Source: CAD feature listing. Evaluate the final solid. Frame: model axes, mm. Round coordinates to 2 decimals unless told otherwise and drop trailing zeros. Order: outer loops, then holes, each group sorted by start corner. A loop starts at its lowest first (then second) coordinate and runs counter-clockwise, first axis right, second up. Notation, with made-up numbers: (78.5, 47) -> (87.5, 47) arc R14 ccw to (87.5, 74) -> close; hole circle Ø11 at (86.5, -7). An arc over 180 degrees is marked (long way). Use a Markdown table: item, result. Add a question column.
```python
from build123d import *

# Parameters (mm, degrees)
SKETCH2_R           = 2.5
SKETCH2_R_2         = 2
BOSS_EXTRUDE1_DEPTH = 10
SKETCH4_R           = 1.5
CUT_EXTRUDE3_DEPTH  = 16


with BuildPart() as part:
    # Sketch2 → Boss-Extrude1 (new body)
    with BuildSketch(Plane(origin=(0, 0, 0), x_dir=(1, 0, 0), z_dir=(0, 1, 0))):
        with BuildLine():
            Line((0, 7.5), (100, 7.5))
            ThreePointArc((100, 7.5), (107.5, 0), (100, -7.5))
            Line((100, -7.5), (0, -7.5))
            ThreePointArc((0, -7.5), (-7.5, 0), (0, 7.5))
        make_face()
        Circle(SKETCH2_R, mode=Mode.SUBTRACT)
        with Locations((100, 0)):
            Circle(SKETCH2_R_2, mode=Mode.SUBTRACT)
    extrude(amount=BOSS_EXTRUDE1_DEPTH)

    # Sketch4 → Cut-Extrude3 (cut, through all)
    with BuildSketch(Plane(origin=(0, 0, -7.5), x_dir=(-1, 0, 0), z_dir=(0, 0, -1))):
        with Locations((0, 5)):
            Circle(SKETCH4_R)
    extrude(amount=-CUT_EXTRUDE3_DEPTH, mode=Mode.SUBTRACT)


solid = part.part
```
1) Section D-D on z = 5. Output: boundary loops of the cut face in (x, y), then the cut area to 3 significant figures.
2) Section C-C on z = -4.5. Output: boundary loops of the cut face in (x, y).
3) Draft query along Z for faces 1 (the cylindrical face through (1.5, 5.07, -4.79)), 2 (the cylindrical face through (-7.5, 4.93, 0.16)), 3 (the cylindrical face through (2.31, 4.93, 0.96)). Return one class per face: pulls with the +Z half, pulls with the -Z half, needs draft (parallel to the pull), parting line crosses it, or undercut.
4) Section B-B on y = 5. Output: boundary loops of the cut face in (x, z), then the cut area to 3 significant figures.
5) Section A-A on z = 0. Output: boundary loops of the cut face in (x, y).
6) Line query: probe 1 along X at (y, z) = (5, 0); probe 2 along Z at (x, y) = (100, 7.75); probe 3 along Y at (x, z) = (0, 5.3). Output: solid intervals per line, ascending. Write a range as from..to.
7) First-contact query: pin 1 Ø1 at (y, z) = (2, -2) entering from +X; pin 2 Ø4 at (y, z) = (4, -5.5) entering from +X; pin 3 Ø1 at (y, z) = (5, 3) entering from +X. Flat tips, straight axial feed; report the tip coordinate or a pass-through.
Conclusion:
| question | item | result |
|---|---|---|
| 1 | outline | (-5.59, 0) -> (105.59, 0) -> (105.59, 10) -> (-5.59, 10) -> close; hole circle Ø3 at (0, 5) |
| 1 | area | 1,100 mm^2 |
| 2 | outline | (-6, 0) -> (106, 0) -> (106, 10) -> (-6, 10) -> close; hole circle Ø3 at (0, 5) |
| 3 | face 1 | needs draft |
| 3 | face 2 | parting line crosses it |
| 3 | face 3 | undercut |
| 4 | outline | (-1.5, -7.35) -> (-1.5, -2) arc R2.5 cw to (-1.5, 2) -> (-1.5, 7.35) arc R7.5 ccw to start; (1.5, -7.5) -> (100, -7.5) arc R7.5 ccw to (100, 7.5) -> (1.5, 7.5) -> (1.5, 2) arc R2.5 cw to (1.5, -2) -> close; hole circle Ø4 at (100, 0) |
| 4 | area | 1,610 mm^2 |
| 5 | outline | (-7.5, 0) -> (-2.5, 0) -> (-2.5, 10) -> (-7.5, 10) -> close; (2.5, 0) -> (98, 0) -> (98, 10) -> (2.5, 10) -> close; (102, 0) -> (107.5, 0) -> (107.5, 10) -> (102, 10) -> close |
| 6 | probe 1 | x = -7.5..-2.5, 2.5..98, 102..107.5 |
| 6 | probe 2 | z = -7.5..-2, 2..7.5 |
| 6 | probe 3 | y = 0..3.5, 6.5..10 |
| 7 | pin 1 | stops at x = 107.35 |
| 7 | pin 2 | stops at x = 106.63 |
| 7 | pin 3 | stops at x = 107.07 |
